Geometry: final body of the model. Coordinates: model frame, mm. A direction names the side the tool comes from. Coordinates: 2 decimals unless noted, no trailing zeros. Write each loop counter-clockwise with the first axis right and the second up, starting at its lowest first coordinate (ties: lowest second). Pieces come first, ordered by that corner, then holes.
from build123d import *

# Parameters (mm, degrees)
SKETCH1_R           = 1.778
SKETCH1_R_2         = 3.175
BOSS_EXTRUDE1_DEPTH = 5.461


with BuildPart() as part:
    # Sketch1 → Boss-Extrude1 (new body)
    with BuildSketch(Plane(origin=(0, 0, 0), x_dir=(1, 0, 0), z_dir=(0, 1, 0))):
        with BuildLine():
            Line((-35.671169379, 16.048164087), (-13.499793526, -0.074664302))
            ThreePointArc((-13.499793526, -0.074664302), (7.44200849, -11.263503435), (5.363638877, 12.388760148))
            Line((5.363638877, 12.388760148), (-34.259632886, 29.543416329))
            ThreePointArc((-34.259632886, 29.543416329), (-39.855484626, 29.811728531), (-44.234733225, 26.317772344))
            ThreePointArc((-44.234733225, 26.317772344), (-45.865213893, 23.360627542), (-47.298283286, 20.302934833))
            ThreePointArc((-47.298283286, 20.302934833), (-47.541465806, 19.100109045), (-47.282683039, 17.900542834))
            Line((-47.282683039, 17.900542834), (-46.773518475, 16.755633062))
            ThreePointArc((-46.773518475, 16.755633062), (-45.359998522, 15.22299407), (-43.306077078, 14.864626044))
            Line((-43.306077078, 14.864626044), (-35.671169379, 16.048164087))
        make_face()
        with Locations((-20.862458922, 15.093717491)):
            Circle(SKETCH1_R, mode=Mode.SUBTRACT)
        Circle(SKETCH1_R_2, mode=Mode.SUBTRACT)
        with Locations((-37.413253893, 22.259284205)):
            Circle(SKETCH1_R, mode=Mode.SUBTRACT)
    extrude(amount=BOSS_EXTRUDE1_DEPTH)


solid = part.part
Item 1: Pull-direction query (Z, two-part tool) for faces 1 (the cylindrical face through (-0.69, 2.69, 3.1)), 2 (the flat face through (-14.171, 2.692, -20.846)), 3 (the flat face through (-11, 5.461, -9)), 4 (the cylindrical face through (7.1, 2.69, 11.48)); classes: released by +Z, released by -Z, zero draft, split by the parting line, or undercut.
Derived:
face 1: undercut
face 2: released by -Z
face 3: zero draft
face 4: split by the parting line
Item 2: Section D-D, the plane z = 8.5. Output: boundary loops of the cut face in (x, y).
Derived:
outline: (-10.49, 0) - (10.49, 0) - (10.49, 5.46) - (-10.49, 5.46) - close
Item 3: Section A-A, the plane z = 2. Output: boundary loops of the cut face in (x, y).
Derived:
outline: (-13.35, 0) - (-2.47, 0) - (-2.47, 5.46) - (-13.35, 5.46) - close; (2.47, 0) - (13.35, 0) - (13.35, 5.46) - (2.47, 5.46) - close
Item 4: Material intervals for probe 1 along Z at (x, y) = (2.5, 1.2); probe 2 along Z at (x, y) = (-20, 2.75); probe 3 along X at (y, z) = (2.3, 1), sorted ascending.
Derived:
probe 1: z = -13.63 to -1.96, 1.96 to 13.27
probe 2: z = -23.37 to -16.65, -13.54 to -4.65
probe 3: x = -13.46 to -3.01, 3.01 to 13.46
Item 5: Section B-B, the plane x = 0. Output: boundary loops of the cut face in (y, z) (3 decimals).
Derived:
outline: (0, -14.711) - (5.461, -14.711) - (5.461, -3.175) - (0, -3.175) - close; (0, 3.175) - (5.461, 3.175) - (5.461, 13.5) - (0, 13.5) - close
Item 6: Section C-C, the plane y = 4.5. State how many separate pieces and enclosed holes the cut face has, plus the area to 3 significant figures.
Derived:
separate pieces: 1
enclosed holes: 3
area: 1,150 mm2
Item 7: Set-up query: faces 5 (the cylindrical face through (-20.042, 2.692, -13.516)), 6 (the flat face through (-39.54, 2.69, -15.45)). Return all of +Z, -Z, +X, -X, +Y, -Y with unobstructed straight access to the full face (end or side cutting, diameter ignored); none if empty.
Derived:
face 5: +Y, -Y
face 6: +Z, +Y, -Y
Item 8: Pin query (flat end, axial travel): pin 1 (2 mm diameter, centred on x = -32.5, y = 2.5, fed in from -Z); pin 2 (2 mm diameter, centred on x = -1.5, y = 1.5, fed in from -Z). Return the tip coordinate at first contact, or that it passes through.
Derived:
pin 1: stops at z = -29.21
pin 2: stops at z = -15.79
